The listing builds one solid part. Answer for the finished solid, in the listing's coordinates (mm). Face numbers are marked on the shaded views. Coordinates: 2 decimals unless noted, no trailing zeros. Order: outer loops, then holes, each group sorted by start corner. A loop starts at its lowest first (then second) coordinate and runs counter-clockwise, first axis right, second up. Notation, with made-up numbers: (47.5, -32) -> (91.5, -32) arc R21 cw to (91.5, -8) -> close; hole circle Ø2 at (50.25, 64). An arc over 180 degrees is marked (long way). Answer in a Markdown table with one row per item.
```python
from build123d import *

# Parameters (mm, degrees)
SKETCH1_R           = 255.21412
SKETCH1_R_2         = 254
BOSS_EXTRUDE1_DEPTH = 508
SKETCH3_R           = 15.875
CUT_EXTRUDE1_DEPTH  = 304.8


with BuildPart() as part:
    # Sketch1 → Boss-Extrude1 (new body)
    with BuildSketch(Plane(origin=(0, 0, 0), x_dir=(1, 0, 0), z_dir=(0, 1, 0))):
        Circle(SKETCH1_R)
        Circle(SKETCH1_R_2, mode=Mode.SUBTRACT)
    extrude(amount=BOSS_EXTRUDE1_DEPTH)

    # Sketch2 → Revolve1 (revolve)
    with BuildSketch(Plane.XY):
        Polygon((254, 0), (38.989, -372.409976186), (40.20312, -372.409976186), (255.21412, 0), align=None)
    revolve(axis=Axis((0, -439.940905122, 0), (0, 1, 0)))

    # Sketch3 → Cut-Extrude1 (cut)
    with BuildSketch(Plane(origin=(0, 53.975, 0), x_dir=(0, 0, -1), z_dir=(1, 0, 0))):
        with Locations((-57.15, 384.980800527)):
            Circle(SKETCH3_R)
    extrude(amount=-CUT_EXTRUDE1_DEPTH, mode=Mode.SUBTRACT)


solid = part.part
```
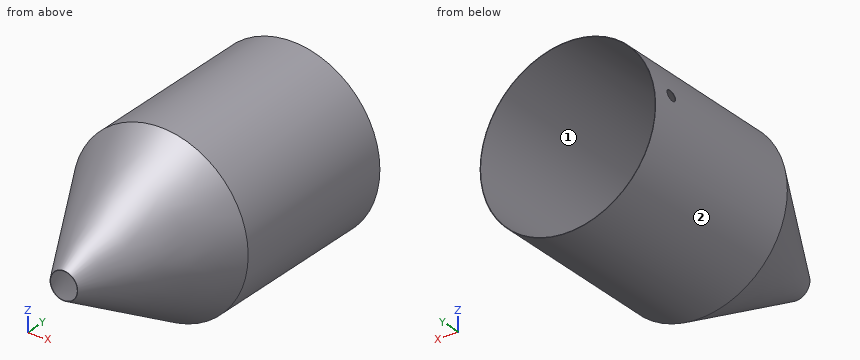
(1) A cutting plane is placed at C-C, the plane y = 211.5. Determine the outline of the cut face in (x, z), then the cut area to 3 significant figures.
Check values:
| item | result |
|---|---|
| outline | circle Ø510.43 at (0, 0); hole circle Ø508 at (0, 0) |
| area | 1,940 mm² |
(2) Find the intervals of material crossed by line 1 along Z through (x, y) = (0, 309.5); line 2 along X through (y, z) = (46, 220), in increasing order. Write a range as from..to.
Check values:
| item | result |
|---|---|
| line 1 | -255.21..-254, 254..255.21 |
| line 2 | -129.36..-126.95, 126.95..129.36 |
(3) For a pull along X with two mould halves and no side action, classify the marked faces 1 and 2 as released by +X, released by -X, zero draft, split by the parting line, or undercut.
Check values:
| item | result |
|---|---|
| face 1 | undercut |
| face 2 | split by the parting line |
(4) A cutting plane is placed at D-D, the plane y = -181. Determine the outline of the cut face in (x, z), then the cut area to 3 significant figures.
Check values:
| item | result |
|---|---|
| outline | circle Ø301.43 at (0, 0); hole circle Ø299 at (0, 0) |
| area | 1,150 mm² |
(5) A cutting plane is placed at A-A, the plane x = 0. Determine the outline of the cut face in (y, z).
Check values:
| item | result |
|---|---|
| outline | (-372.41, -40.2) -> (0, -255.21) -> (508, -255.21) -> (508, -254) -> (0, -254) -> (-372.41, -38.99) -> close; (-372.41, 38.99) -> (0, 254) -> (508, 254) -> (508, 255.21) -> (0, 255.21) -> (-372.41, 40.2) -> close |
(6) Flat-ended cylindrical pins translate along their axes: pin 1 (6 mm diameter, centred on y = 245, z = -29, fed in from +X); pin 2 (6 mm diameter, centred on y = 63.5, z = 52.5, fed in from +X); pin 3 (3 mm diameter, centred on y = 289.5, z = 131.5, fed in from +X); pin 4 (6 mm diameter, centred on x = 34, z = 7.5, fed in from +Y). Find the tip coordinate at first contact, or state that the pin passes through.
Check values:
| item | result |
|---|---|
| pin 1 | x = 253.89 |
| pin 2 | x = 250.37 |
| pin 3 | x = 219.62 |
| pin 4 | through |
(7) A cutting plane is placed at B-B, the plane z = 0. Determine the outline of the cut face in (x, y), then the cut area to 3 significant figures.
Check values:
| item | result |
|---|---|
| outline | (-255.21, 0) -> (-40.2, -372.41) -> (-38.99, -372.41) -> (-254, 0) -> (-254, 508) -> (-255.21, 508) -> close; (38.99, -372.41) -> (40.2, -372.41) -> (255.21, 0) -> (255.21, 508) -> (254, 508) -> (254, 0) -> close |
| area | 2,140 mm² |
